Design review of the part built by this model. Coordinates are the model's own, in mm. Face numbers are marked on the shaded views. A direction names the side the tool comes from. Give positions to 0.01 mm unless a question says otherwise; leave off trailing zeros. Loops run counter-clockwise (first coordinate to the right, second up) from the corner with the lowest first, then second, coordinate; pieces in that order, holes last. Notation, with made-up numbers: M -33,81.5 L -12,81.5 A20 cw -12,100.5 Z; hole C 63.25,14.5 d3. An arc over 180 degrees is marked long. Use a Markdown table: item, result. Add a question column.
(1) Add section C-C, the plane y = -59. Give the boundary of the cut face in (x, z), then the cut area to 3 significant figures.
(2) For probe 1 along X at (y, z) = (-68.75, -30.5); probe 2 along Z at (x, y) = (47, -68); probe 3 along Z at (x, y) = (47.5, -67.5), list the stretches that pass through material, from the lowest coordinate up.
(3) Add section A-A, the plane x = 0. Give the boundary of the cut face in (y, z).
(4) Draft analysis for pull direction X (two halves, no side actions). For the marked faces 1, 2 and 3, state which applies: pulls with the +X half, pulls with the -X half, needs draft (parallel to the pull), parting line crosses it, or undercut.
(5) Add section B-B, the plane y = -41.8. Give the boundary of the cut face in (x, z), then the cut area to 3 significant figures.
(6) Add section D-D, the plane z = -7. Give the boundary of the cut face in (x, y), then the cut area to 3 significant figures.
(7) Insertion check: pin 1 Ø6 at (x, z) = (-47.5, -30.5) entering from -Y; pin 2 Ø1.5 at (x, z) = (-24.5, -36.5) entering from +Y; pin 3 Ø13.5 at (x, y) = (-2.5, -43.5) entering from -Z; pin 4 Ø12 at (x, y) = (19.5, -45.5) entering from -Z. Each pin has a flat end and moves straight along its axis. Give the tip position at first contact, or say it passes through.
(8) For the marked faces 4 and 5, list the 3-axis set-ups (+Z, -Z, +X, -X, +Y, -Y) from which the entire face can be reached by the end or side of a thin tool; tool diameter is ignored.
```python
from build123d import *

# Parameters (mm, degrees)
SKETCH_1_W          = 120
SKETCH_1_H          = 60
EXTRUDE_1_DEPTH     = 62
SKETCH_3_W          = 120
SKETCH_3_H          = 50
CUT_EXTRUDE_1_DEPTH = 40
CUT_EXTRUDE_2_DEPTH = 121
CUT_EXTRUDE_3_DEPTH = 50
SKETCH_7_R          = 12
CUT_EXTRUDE_4_DEPTH = 50
SKETCH_8_W          = 120
SKETCH_8_H          = 10
CUT_EXTRUDE_5_DEPTH = 10
FILLET_1_R          = 10
FILLET_2_R          = 10
FILLET_3_R          = 10
SKETCH_9_R          = 2.5
CUT_EXTRUDE_6_DEPTH = 10


with BuildPart() as part:
    # 草图1 → 凸台-拉伸1 (new body)
    with BuildSketch(Plane(origin=(0, -10, 0), x_dir=(1, 0, 0), z_dir=(0, 1, 0))):
        with Locations((0, 32.5)):
            Rectangle(SKETCH_1_W, SKETCH_1_H)
    extrude(amount=-EXTRUDE_1_DEPTH)

    # 草图3 → 切除-拉伸1 (cut)
    with BuildSketch(Plane(origin=(0, -10, 0), x_dir=(1, 0, 0), z_dir=(0, 1, 0))):
        with Locations((0, 37.5)):
            Rectangle(SKETCH_3_W, SKETCH_3_H)
    extrude(amount=-CUT_EXTRUDE_1_DEPTH, mode=Mode.SUBTRACT)

    # 草图4 → 切除-拉伸2 (cut, through all)
    with BuildSketch(Plane(origin=(60, 0, 0), x_dir=(0, 0, -1), z_dir=(1, 0, 0))):
        with BuildLine():
            Line((27.5, -65), (62.5, -65))
            Line((62.5, -65), (62.5, -50))
            Line((62.5, -50), (12.5, -50))
            ThreePointArc((12.5, -50), (16.893398282, -60.606601718), (27.5, -65))
        make_face()
    extrude(amount=-CUT_EXTRUDE_2_DEPTH, mode=Mode.SUBTRACT)

    # 草图6 → 切除-拉伸3 (cut, symmetric)
    with BuildSketch(Plane(origin=(0, 0, 0), x_dir=(0, 0, -1), z_dir=(1, 0, 0))):
        Polygon((12.5, -50), (12.5, -65), (27.5, -65), align=None)
    extrude(amount=CUT_EXTRUDE_3_DEPTH, both=True, mode=Mode.SUBTRACT)

    # 草图7 → 切除-拉伸4 (cut, symmetric)
    with BuildSketch(Plane(origin=(0, 0, -12.5), x_dir=(-1, 0, 0), z_dir=(0, 0, -1))):
        with Locations((0, -41.8)):
            Circle(SKETCH_7_R)
    extrude(amount=CUT_EXTRUDE_4_DEPTH, both=True, mode=Mode.SUBTRACT)

    # 草图8 → 切除-拉伸5 (cut)
    with BuildSketch(Plane(origin=(0, -10, 0), x_dir=(1, 0, 0), z_dir=(0, 1, 0))):
        with Locations((0, 7.5)):
            Rectangle(SKETCH_8_W, SKETCH_8_H)
    extrude(amount=-CUT_EXTRUDE_5_DEPTH, mode=Mode.SUBTRACT)

    # 圆角1
    fillet_1_edges = [part.edges().sort_by_distance(p)[0] for p in [
        (60, -20, -7.5),
        (-60, -20, -7.5),
    ]]
    fillet(fillet_1_edges, radius=FILLET_1_R)

    # 圆角2
    fillet_2_edges = [part.edges().sort_by_distance(p)[0] for p in [
        (-60, -68.5, -62.5),
        (60, -68.5, -62.5),
    ]]
    fillet(fillet_2_edges, radius=FILLET_2_R)

    # 圆角3
    fillet_3_edges = [part.edges().sort_by_distance(p)[0] for p in [
        (0, -72, -2.5),
    ]]
    fillet(fillet_3_edges, radius=FILLET_3_R)

    # 草图9 → 切除-拉伸6 (cut)
    with BuildSketch(Plane(origin=(0, -65, 0), x_dir=(1, 0, 0), z_dir=(0, 1, 0))):
        with Locations((47.5, 50.5)):
            Circle(SKETCH_9_R)
        with Locations((47.5, 30.5)):
            Circle(SKETCH_9_R)
        with Locations((-47.5, 50.5)):
            Circle(SKETCH_9_R)
        with Locations((-47.5, 30.5)):
            Circle(SKETCH_9_R)
    extrude(amount=-CUT_EXTRUDE_6_DEPTH, mode=Mode.SUBTRACT)


solid = part.part
```
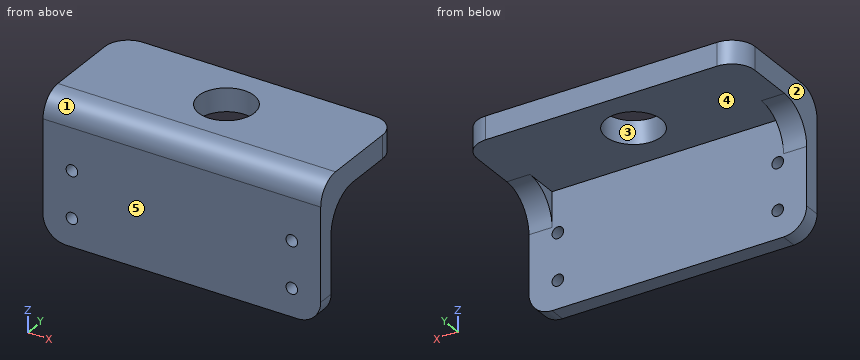
Established:
| question | item | result |
|---|---|---|
| 1 | outline | M -60,-15.5 L -50,-15.5 L -50,-12.5 L 50,-12.5 L 50,-15.5 L 60,-15.5 L 60,-2.5 L -60,-2.5 Z |
| 1 | area | 1,260 mm^2 |
| 2 | probe 1 | -60 to -50, -45 to 45, 50 to 60 |
| 2 | probe 2 | -62.5 to -52.95, -48.05 to -32.95, -28.05 to -4.5 |
| 2 | probe 3 | -62.5 to -53, -48 to -33, -28 to -4.15 |
| 3 | outline | M -72,-62.5 L -65,-62.5 L -65,-12.5 L -53.8,-12.5 L -53.8,-2.5 L -62,-2.5 A10 ccw -72,-12.5 Z; M -29.8,-12.5 L -20,-12.5 L -20,-2.5 L -29.8,-2.5 Z |
| 4 | face 1 | needs draft |
| 4 | face 2 | pulls with the -X half |
| 4 | face 3 | undercut |
| 5 | outline | M -60,-12.5 L -12,-12.5 L -12,-2.5 L -60,-2.5 Z; M 12,-12.5 L 60,-12.5 L 60,-2.5 L 12,-2.5 Z |
| 5 | area | 960 mm^2 |
| 6 | outline | M -60,-70.35 L 60,-70.35 L 60,-30 A10 ccw 50,-20 L -50,-20 A10 ccw -60,-30 Z; hole C 0,-41.8 d24 |
| 6 | area | 5,550 mm^2 |
| 7 | pin 1 | y = -72 |
| 7 | pin 2 | y = -65 |
| 7 | pin 3 | through |
| 7 | pin 4 | z = -12.5 |
| 8 | face 4 | -Z, +Y |
| 8 | face 5 | +Z, -Z, +X, -X, -Y |
